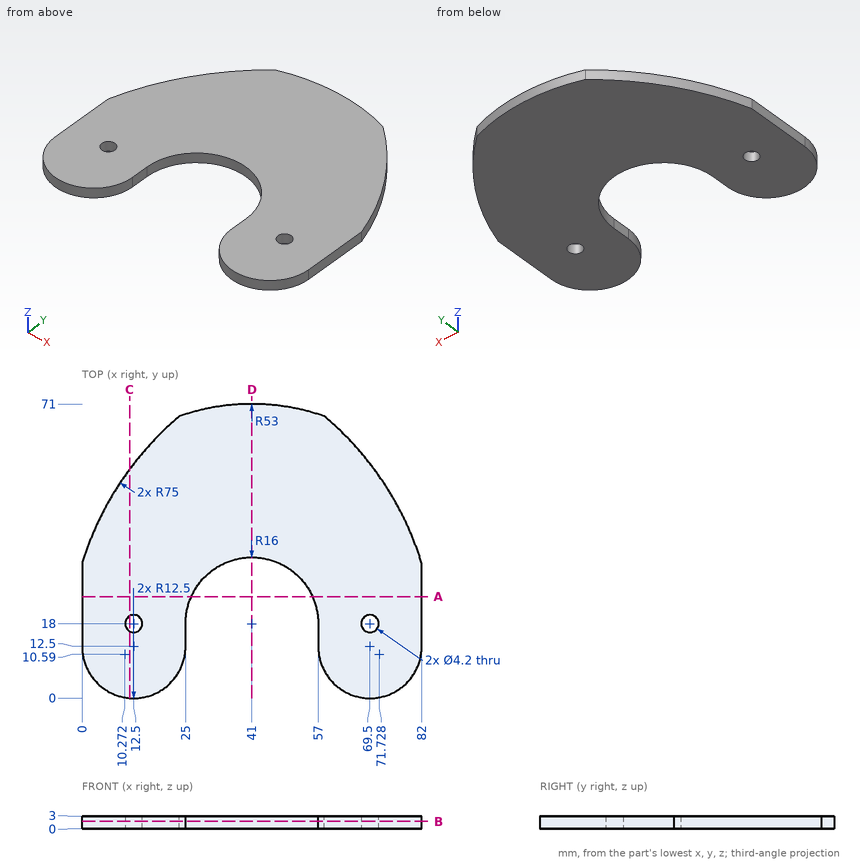
Source: three-view drawing plus pictorial views. Frame: mm from the lowest corner of the part. Give positions to 0.01 mm unless a question says otherwise; leave off trailing zeros. Loops run counter-clockwise (first coordinate to the right, second up) from the corner with the lowest first, then second, coordinate; pieces in that order, holes last. Notation, with made-up numbers: (57.25, 13.5) -> (95.25, 13.5) arc R15 ccw to (95.25, 27.5) -> close; hole circle Ø11 at (5.5, -31). An arc over 180 degrees is marked (long way). Put each result on its own line as item: value. Start each with the question number.
1) Contact query for a flat-ended pin moving along its axis: P1, Ø8, axis at x = 34, y = 22, coming from the +Z side. Output: stop coordinate, or through.
2) Cut plane A-A (y = 24.5). Return loops of the section in (x, z).
3) Cut plane D-D (x = 41). Return loops of the section in (y, z), then the cut area to 3 significant figures.
4) Cut plane C-C (x = 11.5). Return loops of the section in (y, z) (1 decimal), then the cut area to 3 significant figures.
5) Material intervals for probe 1 along X at (y, z) = (19, 0.2) (1 decimal); probe 2 along X at (y, z) = (15.5, 2.4); probe 3 along Y at (x, z) = (12.5, 1.05), sorted ascending.
6) Cut plane B-B (z = 1.75). Return loops of the section in (x, y).
Results are:
1. P1: passes through
2. outline: (0, 0) -> (26.38, 0) -> (26.38, 3) -> (0, 3) -> close; (55.62, 0) -> (82, 0) -> (82, 3) -> (55.62, 3) -> close
3. outline: (34, 0) -> (71, 0) -> (71, 3) -> (34, 3) -> close
3. area: 111 mm2
4. outline: (0, 0) -> (16.2, 0) -> (16.2, 3) -> (0, 3) -> close; (19.8, 0) -> (55.3, 0) -> (55.3, 3) -> (19.8, 3) -> close
4. area: 155 mm2
5. probe 1: x = 0 to 10.7, 14.3 to 25, 57 to 67.7, 71.3 to 82
5. probe 2: x = 0 to 25, 57 to 82
5. probe 3: y = 0 to 15.9, 20.1 to 56.6
6. outline: (0, 12.5) arc R12.5 ccw to (25, 12.5) -> (25, 18) arc R16 cw to (57, 18) -> (57, 12.5) arc R12.5 ccw to (82, 12.5) -> (82, 32.5) arc R75 ccw to (58.5, 68.03) arc R53 ccw to (23.5, 68.03) arc R75 ccw to (0, 32.5) -> close; hole circle Ø4.2 at (12.5, 18); hole circle Ø4.2 at (69.5, 18)
